Verification items for the finished model (mm, model axes). Face numbers are marked on the shaded views. A direction names the side the tool comes from. Round coordinates to 2 decimals unless told otherwise and drop trailing zeros. Order: outer loops, then holes, each group sorted by start corner. A loop starts at its lowest first (then second) coordinate and runs counter-clockwise, first axis right, second up. Notation, with made-up numbers: M 33.25,-21.75 L 86.25,-21.75 A7 cw 86.25,-16.75 Z; hole C -5,34.5 d1. An arc over 180 degrees is marked long. Answer as a JSON object with one key per item and string values. Group by question number.
```python
from build123d import *

# Parameters (mm, degrees)
BOSS_EXTRUDE1_DEPTH = 5


with BuildPart() as part:
    # Sketch1 → Boss-Extrude1 (new body)
    with BuildSketch(Plane.XY):
        Polygon((-10, 30), (-15, 30), (-15, -30), (-10, -30), (-10, -35), (-5, -35), (-5, -30), (-1.5, -30), (-1.5, -27), (-2.6, -27), (-2.6, -24.7), (-1.5, -24.7), (-1.5, -20), (1.5, -20), (1.5, -24.7), (2.6, -24.7), (2.6, -27), (1.5, -27), (1.5, -30), (5, -30), (5, -35), (10, -35), (10, -30), (15, -30), (15, 30), (10, 30), (10, 35), (5, 35), (5, 30), (1.5, 30), (1.5, 27), (2.6, 27), (2.6, 24.7), (1.5, 24.7), (1.5, 20), (-1.5, 20), (-1.5, 24.7), (-2.6, 24.7), (-2.6, 27), (-1.5, 27), (-1.5, 30), (-5, 30), (-5, 35), (-10, 35), align=None)
        with BuildLine():
            ThreePointArc((-4.156470727, -15), (-6.656470727, -17.5), (-9.156470727, -15))
            Line((-9.156470727, -15), (-9.156470727, -5))
            ThreePointArc((-9.156470727, -5), (-6.656470727, -2.5), (-4.156470727, -5))
            Line((-4.156470727, -5), (-4.156470727, -15))
        make_face(mode=Mode.SUBTRACT)
        with BuildLine():
            Line((9.156470727, -5), (9.156470727, -15))
            ThreePointArc((9.156470727, -15), (6.656470727, -17.5), (4.156470727, -15))
            Line((4.156470727, -15), (4.156470727, -5))
            ThreePointArc((4.156470727, -5), (6.656470727, -2.5), (9.156470727, -5))
        make_face(mode=Mode.SUBTRACT)
        with BuildLine():
            Line((-9.156470727, 5), (-9.156470727, 15))
            ThreePointArc((-9.156470727, 15), (-6.656470727, 17.5), (-4.156470727, 15))
            Line((-4.156470727, 15), (-4.156470727, 5))
            ThreePointArc((-4.156470727, 5), (-6.656470727, 2.5), (-9.156470727, 5))
        make_face(mode=Mode.SUBTRACT)
        with BuildLine():
            ThreePointArc((4.156470727, 15), (6.656470727, 17.5), (9.156470727, 15))
            Line((9.156470727, 15), (9.156470727, 5))
            ThreePointArc((9.156470727, 5), (6.656470727, 2.5), (4.156470727, 5))
            Line((4.156470727, 5), (4.156470727, 15))
        make_face(mode=Mode.SUBTRACT)
    extrude(amount=BOSS_EXTRUDE1_DEPTH)


solid = part.part
```
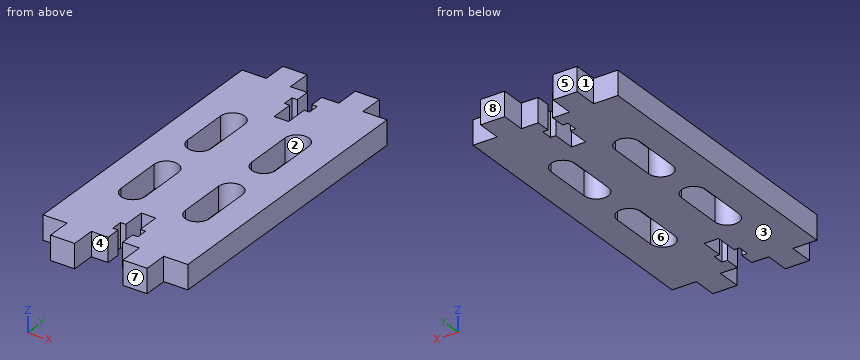
Q1. Tool access check on the marked faces 1, 2, 3, 4 and 5. Record the directions out of +Z, -Z, +X, -X, +Y, -Y that give a thin tool (end or side, any length) a straight path to the whole face; none if there is none.
Q2. Thickness scan on line 1 (Y direction, x = 2, z = 3.7); line 2 (X direction, y = 6, z = 2.2); line 3 (X direction, y = 16, z = 1). Record the ranges inside material, lowest first. Write a range as from..to.
Q3. Gauge pin test, flat ends, axial feed: pin 1 Ø0.6 at (x, z) = (2, 3) entering from +Y; pin 2 Ø2.5 at (x, z) = (12, 3) entering from -Y; pin 3 Ø1.5 at (x, y) = (-6.5, 15.5) entering from -Z. Record the tip position at first contact, or that the pin passes through.
Q4. Cross-section at C-C, the plane x = -13. Record the cut outline in (y, z), then the cut area to 3 significant figures.
Q5. Cross-section at A-A, the plane y = -13. Record the cut outline in (x, z), then the cut area to 3 significant figures.
Q6. Cross-section at D-D, the plane y = -4. Record the cut outline in (x, z).
Q7. Release check for a two-part mould opening along Y. For the marked faces 6, 7 and 8 record: released by +Y, released by -Y, zero draft, split by the parting line, or undercut.
Q8. Cross-section at B-B, the plane z = 3.5. Give the number of separate pieces and of enclosed holes in the cut face, then the cut area to 3 significant figures.
Conclusion:
{
 "1": {"face 1": "+Z, -Z, -X, +Y", "face 2": "+Z, -Z", "face 3": "-Z, +X, -X, +Y, -Y", "face 4": "+Z, -Z, -Y", "face 5": "+Z, -Z, +X, -X, +Y"},
 "2": {"line 1": "-30..-27, -24.7..24.7, 27..30", "line 2": "-15..-9.16, -4.16..4.16, 9.16..15", "line 3": "-15..-8.95, -4.37..4.37, 8.95..15"},
 "3": {"pin 1": "y = 30", "pin 2": "y = -30", "pin 3": "through"},
 "4": {"outline": "M -30,0 L 30,0 L 30,5 L -30,5 Z", "area": "300 mm2"},
 "5": {"outline": "M -15,0 L -9.16,0 L -9.16,5 L -15,5 Z; M -4.16,0 L 4.16,0 L 4.16,5 L -4.16,5 Z; M 9.16,0 L 15,0 L 15,5 L 9.16,5 Z", "area": "100 mm2"},
 "6": {"outline": "M -15,0 L -8.95,0 L -8.95,5 L -15,5 Z; M -4.37,0 L 4.37,0 L 4.37,5 L -4.37,5 Z; M 8.95,0 L 15,0 L 15,5 L 8.95,5 Z"},
 "7": {"face 6": "undercut", "face 7": "released by -Y", "face 8": "released by +Y"},
 "8": {"separate pieces": "1", "enclosed holes": "4", "area": "1,550 mm2"}
}
